For this review, use the dimensioned drawing (mm, ordinates from the lowest corner) and the shaded views. A direction names the side the tool comes from. Give positions to 0.01 mm unless a question says otherwise; leave off trailing zeros. Write each loop counter-clockwise with the first axis right and the second up, starting at its lowest first coordinate (ties: lowest second). Pieces come first, ordered by that corner, then holes. Notation, with made-up numbers: M 21.5,50 L 27.5,50 A16 cw 27.5,61 Z; hole C 87,-20 d11. An arc over 180 degrees is marked long. Write each question's results on one line, items separated by ' | '. Start each with the question number.
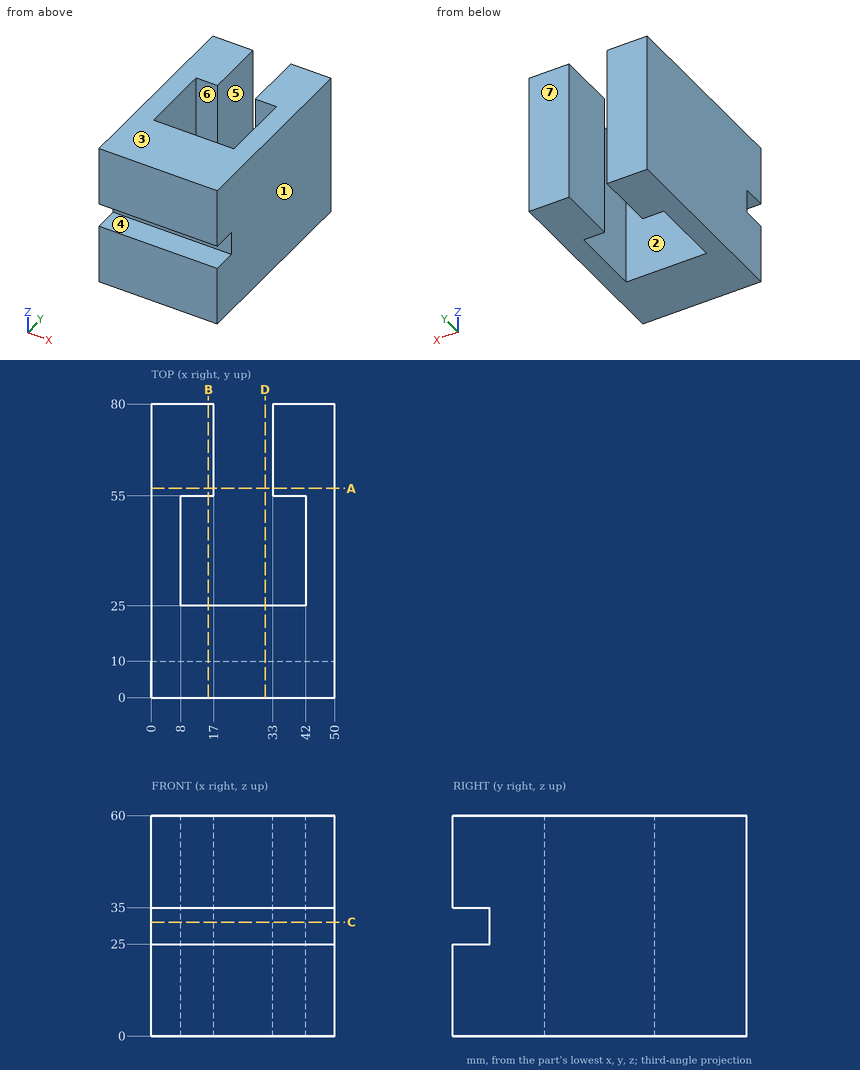
(1) Wall thickness on L1, parallel to X at y = 62, z = 38; L2, parallel to Y at x = 33.5, z = 51; L3, parallel to X at y = 42, z = 23.5: over which ranges is each line inside the solid? List them lowest first.
(2) Add section C-C (z = 31). State the section outline as (x, y) points.
(3) Add section A-A (y = 57). State the section outline as (x, z) points, then the cut area to 3 significant figures.
(4) Add section D-D (x = 31). State the section outline as (y, z) points.
(5) Clearance check with a flat-ended pin moving along its axis: P1, Ø8, axis at x = 23.5, z = 27.5, coming from the +Y side. State where the tip first meets the part, or that it passes through.
(6) Machinability: for the marked faces 4, 5, 6 and 7, which of the approach directions +Z, -Z, +X, -X, +Y, -Y give a long, thin tool a straight path to every point of the face, cutting with its end or side? Answer none if there is none.
(7) Add section B-B (x = 15.5). State the section outline as (y, z) points.
(8) Draft analysis for pull direction X (two halves, no side actions). For the marked faces 1, 2 and 3, state which applies: pulls with the +X half, pulls with the -X half, needs draft (parallel to the pull), parting line crosses it, or undercut.
Calculated:
1) L1: x = 0 to 17, 33 to 50 | L2: y = 0 to 25, 55 to 80 | L3: x = 0 to 8, 42 to 50
2) outline: M 0,10 L 50,10 L 50,80 L 33,80 L 33,55 L 42,55 L 42,25 L 8,25 L 8,55 L 17,55 L 17,80 L 0,80 Z
3) outline: M 0,0 L 17,0 L 17,60 L 0,60 Z; M 33,0 L 50,0 L 50,60 L 33,60 Z | area: 2,040 mm²
4) outline: M 0,0 L 25,0 L 25,60 L 0,60 L 0,35 L 10,35 L 10,25 L 0,25 Z
5) P1: stops at y = 25
6) face 4: +X, -X, -Y | face 5: +Z, -Z, +Y | face 6: +Z, -Z | face 7: +Z, -Z, +X, -X, +Y
7) outline: M 0,0 L 25,0 L 25,60 L 0,60 L 0,35 L 10,35 L 10,25 L 0,25 Z; M 55,0 L 80,0 L 80,60 L 55,60 Z
8) face 1: pulls with the +X half | face 2: undercut | face 3: needs draft
